Part model, mm, in its own coordinate system. A direction names the side the tool comes from. Coordinates: 2 decimals unless noted, no trailing zeros. Loops run counter-clockwise (first coordinate to the right, second up) from the corner with the lowest first, then second, coordinate; pieces in that order, holes last. Notation, with made-up numbers: (35.25, 51.5) - (47.25, 51.5) arc R21 cw to (47.25, 84.5) - close; hole circle Ø1 at (60, 31). An arc over 180 degrees is marked (long way). Use a Markdown table: item, result. Add a question column.
1) Band-saw the part on B-B (x = 6.5). Give the cut face in (y, z), plus the area to 3 significant figures.
2) Band-saw the part on D-D (x = 9.25). Give the cut face in (y, z).
3) Pull direction Y, two halves, no side cores. Call faces 1 (the face through (6, -5, 0)), 2 (the face through (2.908, 0.121, 11.049)), 3 (the face through (0.5, -3.96, 12.32)): +Y half, -Y half, draft (parallel to the pull), parting line (faces both ways), or undercut.
4) Probe probe 1 along Z at (x, y) = (7, -2.5); probe 2 along Y at (x, z) = (3.75, 4.75); probe 3 along X at (y, z) = (-3, 18.5). List the from-to ranges inside material, lowest first. Write a range as [from, to].
5) Band-saw the part on C-C (z = 14). Give the cut face in (x, y), plus the area to 3 significant figures.
6) Drop flat-ended pins along their axis: P1, Ø5, axis at x = 5.65, y = 0, coming from the -Z side; P2, Ø2, axis at x = 4, y = 2.5, coming from the +Z side; P3, Ø4, axis at x = 3.5, y = -1.5, coming from the +Z side; P4, Ø2, axis at y = 3, z = 7, coming from the -X side. Give the stop position or say it passes through.
7) Tool access for faces 4 (the face through (6, -5, 25)), 5 (the face through (10.185, 1.427, 22.288)), 6 (the face through (1.124, 1.427, 3.698)): list every direction of +Z, -Z, +X, -X, +Y, -Y with a clear straight run to the whole face (end or side of a thin tool).
8) Band-saw the part on A-A (y = 0). Give the cut face in (x, z).
from build123d import *

# Parameters (mm, degrees)
SKETCH2_R           = 6.5
BOSS_EXTRUDE1_DEPTH = 25
SKETCH3_R           = 4.75
CUT_EXTRUDE1_DEPTH  = 5.5
SKETCH4_R           = 4.25
CUT_EXTRUDE2_DEPTH  = 5
SKETCH6_R           = 4.75
CUT_EXTRUDE3_DEPTH  = 7.5
CUT_EXTRUDE4_REACH  = 16.5
SKETCH7_R           = 2.75


with BuildPart() as part:
    # Sketch2 → Boss-Extrude1 (new body)
    with BuildSketch(Plane.XY):
        with Locations((5.654843538, 0)):
            Circle(SKETCH2_R)
    extrude(amount=BOSS_EXTRUDE1_DEPTH)

    # Sketch3 → Cut-Extrude1 (cut)
    with BuildSketch(Plane.XY.offset(25)):
        with Locations((5.654843538, 0)):
            Circle(SKETCH3_R)
    extrude(amount=-CUT_EXTRUDE1_DEPTH, mode=Mode.SUBTRACT)

    # Sketch4 → Cut-Extrude2 (cut)
    with BuildSketch(Plane.XY.offset(19.5)):
        with Locations((5.654843538, 0)):
            Circle(SKETCH4_R)
    extrude(amount=-CUT_EXTRUDE2_DEPTH, mode=Mode.SUBTRACT)

    # Sketch6 → Cut-Extrude3 (cut)
    with BuildSketch(Plane(origin=(0, 0, 0), x_dir=(-1, 0, 0), z_dir=(0, 0, -1))):
        with Locations((-5.654843538, 0)):
            Circle(SKETCH6_R)
    extrude(amount=-CUT_EXTRUDE3_DEPTH, mode=Mode.SUBTRACT)

    # Sketch7 → Cut-Extrude4 (cut, up to next)
    with BuildSketch(Plane.XY.offset(14.5), mode=Mode.PRIVATE) as cut_extrude4_sk1:
        with Locations((5.654843538, 0)):
            Circle(SKETCH7_R)
    cut_extrude4_tool1 = extrude(cut_extrude4_sk1.sketch, amount=-CUT_EXTRUDE4_REACH, mode=Mode.PRIVATE) & part.part
    add(cut_extrude4_tool1.solids().sort_by_distance((5.654844, 0, 14.5))[0], mode=Mode.SUBTRACT)


solid = part.part
Answer block:
| question | item | result |
|---|---|---|
| 1 | outline | (-6.44, 0) - (-4.67, 0) - (-4.67, 7.5) - (-2.62, 7.5) - (-2.62, 14.5) - (-4.17, 14.5) - (-4.17, 19.5) - (-4.67, 19.5) - (-4.67, 25) - (-6.44, 25) - close; (2.62, 7.5) - (4.67, 7.5) - (4.67, 0) - (6.44, 0) - (6.44, 25) - (4.67, 25) - (4.67, 19.5) - (4.17, 19.5) - (4.17, 14.5) - (2.62, 14.5) - close |
| 1 | area | 122 mm2 |
| 2 | outline | (-5.42, 0) - (-3.1, 0) - (-3.1, 7.5) - (3.1, 7.5) - (3.1, 0) - (5.42, 0) - (5.42, 25) - (3.1, 25) - (3.1, 19.5) - (2.27, 19.5) - (2.27, 14.5) - (-2.27, 14.5) - (-2.27, 19.5) - (-3.1, 19.5) - (-3.1, 25) - (-5.42, 25) - close |
| 3 | face 1 | draft |
| 3 | face 2 | undercut |
| 3 | face 3 | parting line |
| 4 | probe 1 | [7.5, 14.5] |
| 4 | probe 2 | [-6.21, -4.35], [4.35, 6.21] |
| 4 | probe 3 | [-0.11, 2.64], [8.67, 11.42] |
| 5 | outline | circle Ø13 at (5.65, 0); hole circle Ø5.5 at (5.65, 0) |
| 5 | area | 109 mm2 |
| 6 | P1 | through |
| 6 | P2 | z = 14.5 |
| 6 | P3 | z = 19.5 |
| 6 | P4 | x = -0.53 |
| 7 | face 4 | +Z, +X, -X, +Y, -Y |
| 7 | face 5 | +Z |
| 7 | face 6 | -Z |
| 8 | outline | (-0.85, 0) - (0.9, 0) - (0.9, 7.5) - (2.9, 7.5) - (2.9, 14.5) - (1.4, 14.5) - (1.4, 19.5) - (0.9, 19.5) - (0.9, 25) - (-0.85, 25) - close; (8.4, 7.5) - (10.4, 7.5) - (10.4, 0) - (12.15, 0) - (12.15, 25) - (10.4, 25) - (10.4, 19.5) - (9.9, 19.5) - (9.9, 14.5) - (8.4, 14.5) - close |
